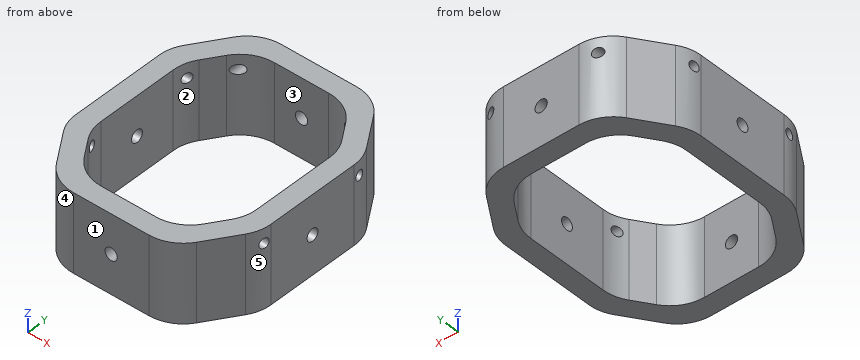
```python
from build123d import *

# Parameters (mm, degrees)
F1_DEPTH  = 25.4
F2_R      = 2.00025
F3_DEPTH  = 39.6875
F4_R      = 2.00025
F5_DEPTH  = 41.275
F6_R      = 12.7
F7_R      = 1.5875
F8_DEPTH  = 25.4
F9_R      = 1.5875
F10_DEPTH = 38.1


with BuildPart() as f1:
    # F0 (on Top) → F1 (new body)
    with BuildSketch(Plane.XY):
        Polygon((31.75, 19.05), (19.05, 38.1), (-19.05, 38.1), (-31.75, 19.05), (-31.75, -19.05), (-19.05, -38.1), (19.05, -38.1), (31.75, -19.05), align=None)
        Polygon((-25.4, -17.1273747004), (-25.4, 17.1273747004), (-15.6515831336, 31.75), (15.6515831336, 31.75), (25.4, 17.1273747004), (25.4, -17.1273747004), (15.6515831336, -31.75), (-15.6515831336, -31.75), align=None, mode=Mode.SUBTRACT)
    extrude(amount=F1_DEPTH)

    # F2 (on Front) → F3 (cut, symmetric)
    with BuildSketch(Plane.XZ):
        with Locations((0, 12.7)):
            Circle(F2_R)
    extrude(amount=F3_DEPTH, both=True, mode=Mode.SUBTRACT)

    # F4 (on Right) → F5 (cut, symmetric)
    with BuildSketch(Plane.YZ):
        with Locations((0, 12.7)):
            Circle(F4_R)
    extrude(amount=F5_DEPTH, both=True, mode=Mode.SUBTRACT)

    # F6
    f6_edges = [f1.edges().sort_by_distance(p)[0] for p in [
        (-25.4, 17.127375, 12.7),
        (-15.651583, 31.75, 12.7),
        (15.651583, 31.75, 12.7),
        (25.4, 17.127375, 12.7),
        (25.4, -17.127375, 12.7),
        (15.651583, -31.75, 12.7),
        (-15.651583, -31.75, 12.7),
        (-25.4, -17.127375, 12.7),
        (-19.05, -38.1, 12.7),
        (-31.75, -19.05, 12.7),
        (19.05, -38.1, 12.7),
        (31.75, -19.05, 12.7),
        (31.75, 19.05, 12.7),
        (19.05, 38.1, 12.7),
        (-19.05, 38.1, 12.7),
        (-31.75, 19.05, 12.7),
    ]]
    fillet(f6_edges, radius=F6_R)

    # F7 (on face) → F8 (cut)
    with BuildSketch(Plane(origin=(0, 38.1, 0), x_dir=(-1, 0, 0), z_dir=(0, 1, 0))):
        with Locations((-17.4625, 20.6375)):
            Circle(F7_R)
        with Locations((17.4625, 20.6375)):
            Circle(F7_R)
    extrude(amount=-F8_DEPTH, mode=Mode.SUBTRACT)

    # F9 (on Right) → F10 (cut, symmetric)
    with BuildSketch(Plane.YZ):
        with Locations((-17.4625, 20.6375)):
            Circle(F9_R)
        with Locations((17.4625, 20.6375)):
            Circle(F9_R)
    extrude(amount=F10_DEPTH, both=True, mode=Mode.SUBTRACT)


solid = f1.part
```
For this review, take the finished solid that the model builds, in its own axes (mm). Face numbers are marked on the shaded views. A direction names the side the tool comes from. Round coordinates to 2 decimals unless told otherwise and drop trailing zeros. Write each loop counter-clockwise with the first axis right and the second up, starting at its lowest first coordinate (ties: lowest second). Pieces come first, ordered by that corner, then holes. Notation, with made-up numbers: M 71.5,-19.75 L 78.5,-19.75 A29 ccw 78.5,8.25 Z; hole C 5.25,73 d11. An arc over 180 degrees is marked long. One line per item, written item: value. Start each with the question number.
(1) We need section D-D (x = -8). Give the boundary of the cut face in (y, z), and give its area (3 significant figures).
(2) Insertion check: pin 1 (1 mm diameter, centred on y = -19.5, z = 8, fed in from +X); pin 2 (3 mm diameter, centred on x = 0, z = 12.7, fed in from -Y); pin 3 (4 mm diameter, centred on y = -17.46, z = 20.64, fed in from -X); pin 4 (3 mm diameter, centred on y = 23.5, z = 13, fed in from +X). Each pin has a flat end and moves straight along its axis. Give the tip position at first contact, or say it passes through.
(3) Wall thickness on line 1 (X direction, y = 7, z = 9); line 2 (Z direction, x = 0, y = 33.5); line 3 (Y direction, x = 6, z = 22.75): over which ranges is each line inside the solid? List them lowest first.
(4) Machinability: for the marked faces 1 and 2, which of the approach directions +Z, -Z, +X, -X, +Y, -Y give a long, thin tool a straight path to every point of the face, cutting with its end or side? Answer none if there is none.
(5) The part is to be moulded in two halves that separate along X. For the marked faces 3, 4 and 5, say which applies: released by +X, released by -X, zero draft, split by the parting line, or undercut.
(6) We need section A-A (x = 0). Give the boundary of the cut face in (y, z), and give its area (3 significant figures).
(7) We need section B-B (y = 0). Give the boundary of the cut face in (x, z).
Result:
1. outline: M -38.1,0 L -31.75,0 L -31.75,25.4 L -38.1,25.4 Z; M 31.75,0 L 38.1,0 L 38.1,25.4 L 31.75,25.4 Z
1. area: 323 mm²
2. pin 1: x = 31.17
2. pin 2: through
2. pin 3: x = -31.75
2. pin 4: x = 29.78
3. line 1: -31.75 to -25.4, 25.4 to 31.75
3. line 2: 0 to 10.7, 14.7 to 25.4
3. line 3: -38.1 to -31.75, 31.75 to 38.1
4. face 1: +Z, -Z, +X, -X, -Y
4. face 2: +Z, -Z
5. face 3: undercut
5. face 4: released by -X
5. face 5: released by +X
6. outline: M -38.1,0 L -31.75,0 L -31.75,10.7 L -38.1,10.7 Z; M -38.1,14.7 L -31.75,14.7 L -31.75,25.4 L -38.1,25.4 Z; M 31.75,0 L 38.1,0 L 38.1,10.7 L 31.75,10.7 Z; M 31.75,14.7 L 38.1,14.7 L 38.1,25.4 L 31.75,25.4 Z
6. area: 272 mm²
7. outline: M -31.75,0 L -25.4,0 L -25.4,10.7 L -31.75,10.7 Z; M -31.75,14.7 L -25.4,14.7 L -25.4,25.4 L -31.75,25.4 Z; M 25.4,0 L 31.75,0 L 31.75,10.7 L 25.4,10.7 Z; M 25.4,14.7 L 31.75,14.7 L 31.75,25.4 L 25.4,25.4 Z
